```python
from build123d import *

# Parameters (mm, degrees)
SKETCH1_W           = 40
SKETCH1_H           = 34
BOSS_EXTRUDE1_DEPTH = 11
SKETCH3_W           = 34
SKETCH3_H           = 20.5
CUT_EXTRUDE1_DEPTH  = 9.5
FILLET2_R           = 1.5
BOSS_EXTRUDE3_DEPTH = 10
FILLET3_R           = 6
FILLET4_R           = 15


with BuildPart() as part:
    # Sketch1 → Boss-Extrude1 (new body)
    with BuildSketch(Plane(origin=(0, 0, 0), x_dir=(1, 0, 0), z_dir=(0, 1, 0))):
        with Locations((20, 17)):
            Rectangle(SKETCH1_W, SKETCH1_H)
    extrude(amount=BOSS_EXTRUDE1_DEPTH)

    # Sketch3 → Cut-Extrude1 (cut)
    with BuildSketch(Plane(origin=(0, 11, 0), x_dir=(1, 0, 0), z_dir=(0, 1, 0))):
        with Locations((20, 17)):
            Rectangle(SKETCH3_W, SKETCH3_H)
    extrude(amount=-CUT_EXTRUDE1_DEPTH, mode=Mode.SUBTRACT)

    # Fillet2
    fillet2_edges = [part.edges().sort_by_distance(p)[0] for p in [
        (3, 6.25, -27.25),
        (3, 6.25, -6.75),
        (37, 6.25, -6.75),
        (37, 6.25, -27.25),
    ]]
    fillet(fillet2_edges, radius=FILLET2_R)

    # Sketch5 → Boss-Extrude3 (add, symmetric)
    with BuildSketch(Plane(origin=(0, 0, -17), x_dir=(-1, 0, 0), z_dir=(0, 0, -1))):
        Polygon((-40, 0), (-52, 0), (-52, 3.5), (-40, 5.5), align=None)
        Polygon((12, 3.5), (0, 5.5), (0, 0), (12, 0), align=None)
    extrude(amount=BOSS_EXTRUDE3_DEPTH, both=True)

    # Fillet3
    fillet3_edges = [part.edges().sort_by_distance(p)[0] for p in [
        (0, 5.5, -34),
        (40, 5.5, -34),
        (40, 5.5, 0),
        (0, 5.5, 0),
    ]]
    fillet(fillet3_edges, radius=FILLET3_R)

    # Fillet4
    # the kernel refuses this fillet: 15 mm, written as the material it adds along each edge
    with BuildSketch(Plane(origin=(0, 29.631189606, -27), x_dir=(0.2922336268554167, 0, -0.9563469597039189), z_dir=(0, -1, 0))) as fillet4_piece_1_section:
        with BuildLine():
            CenterArc((11.524426372, -13.614620328), FILLET4_R, 114.818587472, 48.189685104)
            Line((-2.820778024, -9.231115926), (-4.255298463, -8.792765485))
            Line((-4.255298463, -8.792765485), (-1.43452044, 0.43835044))
            Line((-1.43452044, 0.43835044), (0.43835044, 1.43452044))
            ThreePointArc((0.43835044, 1.43452044), (1.3946974, 1.142286813), (4.598608218, 1.361462033))
            Line((4.598608218, 1.361462033), (5.22822805, 0))
        make_face()
    fillet4_piece_1 = extrude(amount=29.631189606, mode=Mode.PRIVATE)
    fillet4_piece_1 = split(fillet4_piece_1, bisect_by=Plane(origin=(-2.592829237, 5.067861794, -27.668863599), z_dir=(0.16439898730535746, -0.9863939238321437, 0)), keep=Keep.TOP, mode=Mode.PRIVATE)
    add(fillet4_piece_1)
    with BuildSketch(Plane(origin=(0, 29.631189606, -7), x_dir=(0.2922336268554167, 0, 0.9563469597039189), z_dir=(0, -1, 0))) as fillet4_piece_2_section:
        with BuildLine():
            CenterArc((11.524426372, 13.614620328), FILLET4_R, 196.991727423, 48.189685104)
            Line((-2.820778024, 9.231115926), (-4.255298463, 8.792765485))
            Line((-4.255298463, 8.792765485), (-1.43452044, -0.43835044))
            Line((-1.43452044, -0.43835044), (0.43835044, -1.43452044))
            ThreePointArc((0.43835044, -1.43452044), (1.3946974, -1.142286813), (4.598608218, -1.361462033))
            Line((4.598608218, -1.361462033), (5.22822805, 0))
        make_face()
    fillet4_piece_2 = extrude(amount=29.631189606, mode=Mode.PRIVATE)
    fillet4_piece_2 = split(fillet4_piece_2, bisect_by=Plane(origin=(-2.592829237, 5.067861794, -6.331136401), z_dir=(0.16439898730535746, -0.9863939238321437, 0)), keep=Keep.TOP, mode=Mode.PRIVATE)
    add(fillet4_piece_2)
    with BuildSketch(Plane(origin=(40, 29.631189606, -7), x_dir=(-0.29223362685541665, 0, 0.9563469597039189), z_dir=(0, -1, 0))) as fillet4_piece_3_section:
        with BuildLine():
            CenterArc((11.524426372, -13.614620328), FILLET4_R, 114.818587472, 48.189685104)
            Line((-2.820778024, -9.231115926), (-4.255298463, -8.792765485))
            Line((-4.255298463, -8.792765485), (-1.43452044, 0.43835044))
            Line((-1.43452044, 0.43835044), (0.43835044, 1.43452044))
            ThreePointArc((0.43835044, 1.43452044), (1.3946974, 1.142286813), (4.598608218, 1.361462033))
            Line((4.598608218, 1.361462033), (5.22822805, 0))
        make_face()
    fillet4_piece_3 = extrude(amount=29.631189606, mode=Mode.PRIVATE)
    fillet4_piece_3 = split(fillet4_piece_3, bisect_by=Plane(origin=(42.592829237, 5.067861794, -6.331136401), z_dir=(-0.16439898730535732, -0.9863939238321437, 0)), keep=Keep.TOP, mode=Mode.PRIVATE)
    add(fillet4_piece_3)
    with BuildSketch(Plane(origin=(40, 29.631189606, -27), x_dir=(-0.2922336268554167, 0, -0.9563469597039189), z_dir=(0, -1, 0))) as fillet4_piece_4_section:
        with BuildLine():
            CenterArc((11.524426372, 13.614620328), FILLET4_R, 196.991727423, 48.189685104)
            Line((-2.820778024, 9.231115926), (-4.255298463, 8.792765485))
            Line((-4.255298463, 8.792765485), (-1.43452044, -0.43835044))
            Line((-1.43452044, -0.43835044), (0.43835044, -1.43452044))
            ThreePointArc((0.43835044, -1.43452044), (1.3946974, -1.142286813), (4.598608218, -1.361462033))
            Line((4.598608218, -1.361462033), (5.22822805, 0))
        make_face()
    fillet4_piece_4 = extrude(amount=29.631189606, mode=Mode.PRIVATE)
    fillet4_piece_4 = split(fillet4_piece_4, bisect_by=Plane(origin=(42.592829237, 5.067861794, -27.668863599), z_dir=(-0.16439898730535732, -0.9863939238321437, 0)), keep=Keep.TOP, mode=Mode.PRIVATE)
    add(fillet4_piece_4)


solid = part.part
```
Build history of the part. All positions in model axes, mm. A direction names the side the tool comes from. Round coordinates to 2 decimals unless told otherwise and drop trailing zeros. Write each loop counter-clockwise with the first axis right and the second up, starting at its lowest first coordinate (ties: lowest second). Pieces come first, ordered by that corner, then holes. Notation, with made-up numbers: (86, 63) -> (131, 63) arc R22 cw to (131, 85) -> close; hole circle Ø11 at (-28, 27). An arc over 180 degrees is marked (long way). Put each result on its own line as item: value.
Item 1: Slice it at D-D, the plane y = 4.75. Give the cut face in (x, z).
Here are the results:
outline: (-4.5, -27.91) arc R15 cw to (1.53, -32) arc R6 ccw to (6, -34) -> (34, -34) arc R6 ccw to (38.47, -32) arc R15 cw to (44.5, -27.91) -> (44.5, -6.09) arc R15 cw to (38.47, -2) arc R6 ccw to (34, 0) -> (6, 0) arc R6 ccw to (1.53, -2) arc R15 cw to (-4.5, -6.09) -> close; hole (3, -25.75) arc R1.5 ccw to (4.5, -27.25) -> (35.5, -27.25) arc R1.5 ccw to (37, -25.75) -> (37, -8.25) arc R1.5 ccw to (35.5, -6.75) -> (4.5, -6.75) arc R1.5 ccw to (3, -8.25) -> close
Item 2: Wall check: probe 1 along X at (y, z) = (6.25, -22); probe 2 along Z at (x, y) = (17, 6.75); probe 3 along X at (y, z) = (3, -11). Give the ranges that are in metal, low to high. Write a range as from..to.
Here are the results:
probe 1: x = 0..3, 37..40
probe 2: z = -34..-27.25, -6.75..0
probe 3: x = -12..3, 37..52
Item 3: Slice it at A-A, the plane y = 9. Give the cut face in (x, z), plus the area to 3 significant figures.
Here are the results:
outline: (0, -28) arc R6 ccw to (6, -34) -> (34, -34) arc R6 ccw to (40, -28) -> (40, -6) arc R6 ccw to (34, 0) -> (6, 0) arc R6 ccw to (0, -6) -> close; hole (3, -25.75) arc R1.5 ccw to (4.5, -27.25) -> (35.5, -27.25) arc R1.5 ccw to (37, -25.75) -> (37, -8.25) arc R1.5 ccw to (35.5, -6.75) -> (4.5, -6.75) arc R1.5 ccw to (3, -8.25) -> close
area: 634 mm^2
Item 4: Slice it at B-B, the plane x = 18.5. Give the cut face in (y, z).
Here are the results:
outline: (0, -34) -> (11, -34) -> (11, -27.25) -> (1.5, -27.25) -> (1.5, -6.75) -> (11, -6.75) -> (11, 0) -> (0, 0) -> close
Item 5: Tool access for faces 1 (the face through (2.505, 6.799, -1.123)), 2 (the face through (51, 2, -7)), 3 (the face through (40, 8, -17)), 4 (the face through (3, 6, -17)), 5 (the face through (0, 8, -17)): list every direction of +Z, -Z, +X, -X, +Y, -Y with a clear straight run to the whole face (end or side of a thin tool).
Here are the results:
face 1: +Z, -X, +Y
face 2: +Z, +X, +Y, -Y
face 3: +Z, -Z, +X, +Y
face 4: +Y
face 5: +Z, -Z, -X, +Y
Item 6: Slice it at C-C, the plane z = -14.5. Give the cut face in (x, y), plus the area to 3 significant figures.
Here are the results:
outline: (-12, 0) -> (52, 0) -> (52, 3.5) -> (40, 5.5) -> (40, 11) -> (37, 11) -> (37, 1.5) -> (3, 1.5) -> (3, 11) -> (0, 11) -> (0, 5.5) -> (-12, 3.5) -> close
area: 225 mm^2
Item 7: Two-plate mould, pull along Z, no slides. Class faces 6 (the face through (-5.141, 4.643, -17.21)), 7 (the face through (20, 6, -6.75)), 8 (the face through (-11, 2, -7)): pulls with the +Z half, pulls with the -Z half, needs draft (parallel to the pull), parting line crosses it, or undercut.
Here are the results:
face 6: needs draft
face 7: undercut
face 8: pulls with the +Z half
Item 8: Flat gauge pins, fed straight in: P1, Ø0.7, axis at x = 50.5, y = 2, coming from the +Z side; P2, Ø0.7, axis at x = 51.5, y = 1.5, coming from the -Z side; P3, Ø10, axis at x = 15, z = -16, coming from the +Y side. Where does each tip first touch, or does it go through?
Here are the results:
P1: stops at z = -7
P2: stops at z = -27
P3: stops at y = 1.5
